Verification items for this drawing (mm, ordinates from the low corner). A direction names the side the tool comes from. Round coordinates to 2 decimals unless told otherwise and drop trailing zeros. Write each loop counter-clockwise with the first axis right and the second up, starting at its lowest first coordinate (ties: lowest second). Pieces come first, ordered by that corner, then holes. Notation, with made-up numbers: (-36.75, -33) -> (-9.75, -33) arc R8 cw to (-9.75, -20) -> close; hole circle Ø9 at (75, 2). An arc over 180 degrees is marked (long way). One line per item, written item: value.
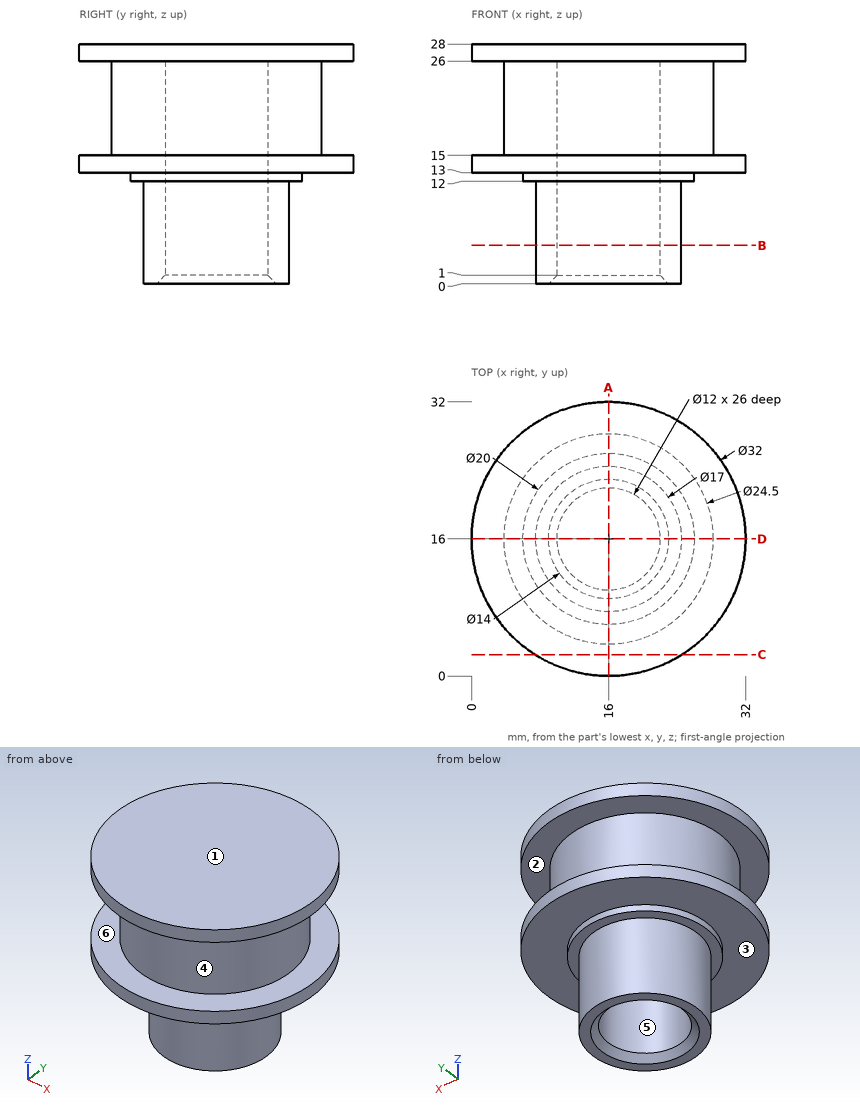
Item 1: Release check for a two-part mould opening along Z. For the marked faces 1, 2, 3 and 4 record: pulls with the +Z half, pulls with the -Z half, needs draft (parallel to the pull), parting line crosses it, or undercut.
Result set:
face 1: pulls with the +Z half
face 2: undercut
face 3: pulls with the -Z half
face 4: undercut
Item 2: Material ranges on line 1 along Y through (x, z) = (16, 8); line 2 along Z through (x, y) = (2.5, 21); line 3 along Y through (x, z) = (16, 20), recorded low to high.
Result set:
line 1: 7.5 to 10, 22 to 24.5
line 2: 13 to 15, 26 to 28
line 3: 3.75 to 10, 22 to 28.25
Item 3: Sectioned sample at B-B (z = 4.5). Enter the section's corners in (x, y), then the cut area to 3 significant figures.
Result set:
outline: circle Ø17 at (16, 16); hole circle Ø12 at (16, 16)
area: 114 mm^2
Item 4: Depth check by flat-ended pin: pin 1 (10 mm diameter, centred on x = 15, y = 14, fed in from -Z); pin 2 (2 mm diameter, centred on y = 12.5, z = 22, fed in from -X); pin 3 (2 mm diameter, centred on x = 27.5, z = 13, fed in from -Y); pin 4 (1 mm diameter, centred on x = 19.5, y = 14.5, fed in from -Z). Enter the tip coordinate at first touch or a pass-through.
Result set:
pin 1: z = 0
pin 2: x = 4.01
pin 3: y = 3.93
pin 4: z = 26
Item 5: Tool access check on the marked faces 5 and 6. Record the directions out of +Z, -Z, +X, -X, +Y, -Y that give a thin tool (end or side, any length) a straight path to the whole face; none if there is none.
Result set:
face 5: -Z
face 6: none
Item 6: Sectioned sample at A-A (x = 16). Enter the section's corners in (y, z).
Result set:
outline: (0, 13) -> (6, 13) -> (6, 12) -> (7.5, 12) -> (7.5, 0) -> (9, 0) -> (10, 1) -> (10, 26) -> (22, 26) -> (22, 1) -> (23, 0) -> (24.5, 0) -> (24.5, 12) -> (26, 12) -> (26, 13) -> (32, 13) -> (32, 15) -> (28.25, 15) -> (28.25, 26) -> (32, 26) -> (32, 28) -> (0, 28) -> (0, 26) -> (3.75, 26) -> (3.75, 15) -> (0, 15) -> close
Item 7: Sectioned sample at C-C (y = 2.5). Enter the section's corners in (x, z).
Result set:
outline: (7.41, 13) -> (24.59, 13) -> (24.59, 15) -> (7.41, 15) -> close; (7.41, 26) -> (24.59, 26) -> (24.59, 28) -> (7.41, 28) -> close
